```python
from build123d import *

# Parameters (mm, degrees)
SKETCH1_R           = 43.55
SKETCH1_R_2         = 42.55
BOSS_EXTRUDE1_DEPTH = 120
CHAMFER1_SIZE       = 10
CHAMFER1_SIZE2      = 0.9
CHAMFER2_SIZE       = 0.9
CHAMFER2_SIZE2      = 10


with BuildPart() as part:
    # Sketch1 → Boss-Extrude1 (new body)
    with BuildSketch(Plane(origin=(0, 0, 0), x_dir=(1, 0, 0), z_dir=(0, 1, 0))):
        Circle(SKETCH1_R)
        Circle(SKETCH1_R_2, mode=Mode.SUBTRACT)
    extrude(amount=BOSS_EXTRUDE1_DEPTH)

    # Chamfer1
    chamfer1_edges = [part.edges().sort_by_distance(p)[0] for p in [
        (-43.55, 120, 0),
    ]]
    chamfer1_side = [part.faces().sort_by_distance(p)[0] for p in [
        (-43.55, 60, 0),
    ]]
    chamfer(chamfer1_edges, length=CHAMFER1_SIZE, length2=CHAMFER1_SIZE2, reference=chamfer1_side[0])

    # Chamfer2
    chamfer2_edges = [part.edges().sort_by_distance(p)[0] for p in [
        (-43.55, 0, 0),
    ]]
    chamfer2_side = [part.faces().sort_by_distance(p)[0] for p in [
        (-43.426821999, 0, 0),
    ]]
    chamfer(chamfer2_edges, length=CHAMFER2_SIZE, length2=CHAMFER2_SIZE2, reference=chamfer2_side[0])


solid = part.part
```
Check sheet for the modelled part. Datum: model origin and axes. Units: mm. Round coordinates to 2 decimals unless told otherwise and drop trailing zeros. Order: outer loops, then holes, each group sorted by start corner. A loop starts at its lowest first (then second) coordinate and runs counter-clockwise, first axis right, second up. Notation, with made-up numbers: (9, 17.5) -> (41, 17.5) arc R24 ccw to (41, 33.5) -> close; hole circle Ø10 at (87, -26). An arc over 180 degrees is marked (long way). Use CSV: the item, a comma, the result in double quotes.
(1) Draft check along X on faces 1 (the face through (-5.573, 1.737, -42.442)), 2 (the face through (-33.766, 59.16, 25.891)). Enter one of: pulls with the +X half, pulls with the -X half, needs draft (parallel to the pull), parting line crosses it, or undercut.
Worked out:
face 1,"parting line crosses it"
face 2,"undercut"
(2) Cross-section at C-C (y = 20). Record the boundary of the cut face in (x, z).
Worked out:
outline,"circle Ø87.1 at (0, 0); hole circle Ø85.1 at (0, 0)"
(3) Cross-section at B-B (z = 0). Record the boundary of the cut face in (x, y), and give its area (3 significant figures).
Worked out:
outline,"(-43.55, 10) -> (-42.65, 0) -> (-42.55, 0) -> (-42.55, 120) -> (-42.65, 120) -> (-43.55, 110) -> close; (42.55, 0) -> (42.65, 0) -> (43.55, 10) -> (43.55, 110) -> (42.65, 120) -> (42.55, 120) -> close"
area,"222 mm²"
(4) Cross-section at A-A (x = 0). Record the boundary of the cut face in (y, z), and give its area (3 significant figures).
Worked out:
outline,"(0, -42.65) -> (10, -43.55) -> (110, -43.55) -> (120, -42.65) -> (120, -42.55) -> (0, -42.55) -> close; (0, 42.55) -> (120, 42.55) -> (120, 42.65) -> (110, 43.55) -> (10, 43.55) -> (0, 42.65) -> close"
area,"222 mm²"
(5) Material ranges on line 1 along Z through (x, y) = (0, 55.5); line 2 along Z through (x, y) = (5, 87), recorded low to high. Write a range as from..to.
Worked out:
line 1,"-43.55..-42.55, 42.55..43.55"
line 2,"-43.26..-42.26, 42.26..43.26"
(6) Depth check by flat-ended pin: pin 1 (4 mm diameter, centred on x = 18, y = 45, fed in from +Z); pin 2 (10 mm diameter, centred on y = 12.5, z = 23.5, fed in from +X); pin 3 (2 mm diameter, centred on x = 12, y = 93, fed in from +Z). Enter the tip coordinate at first touch or a pass-through.
Worked out:
pin 1,"z = 40.5"
pin 2,"x = 39.43"
pin 3,"z = 42.14"
